The figure shows three views and two pictorial views of one solid part (mm, origin at its lowest corner). Answer the questions. A direction names the side the tool comes from. Give positions to 0.01 mm unless a question says otherwise; leave off trailing zeros. Loops run counter-clockwise (first coordinate to the right, second up) from the corner with the lowest first, then second, coordinate; pieces in that order, holes last. Notation, with made-up numbers: M -15.5,-20 L 12.5,-20 A15 ccw 12.5,4 Z; hole C 27,24.5 d1. An arc over 180 degrees is marked long. Answer in a Markdown table with one row per item. Add a question column.
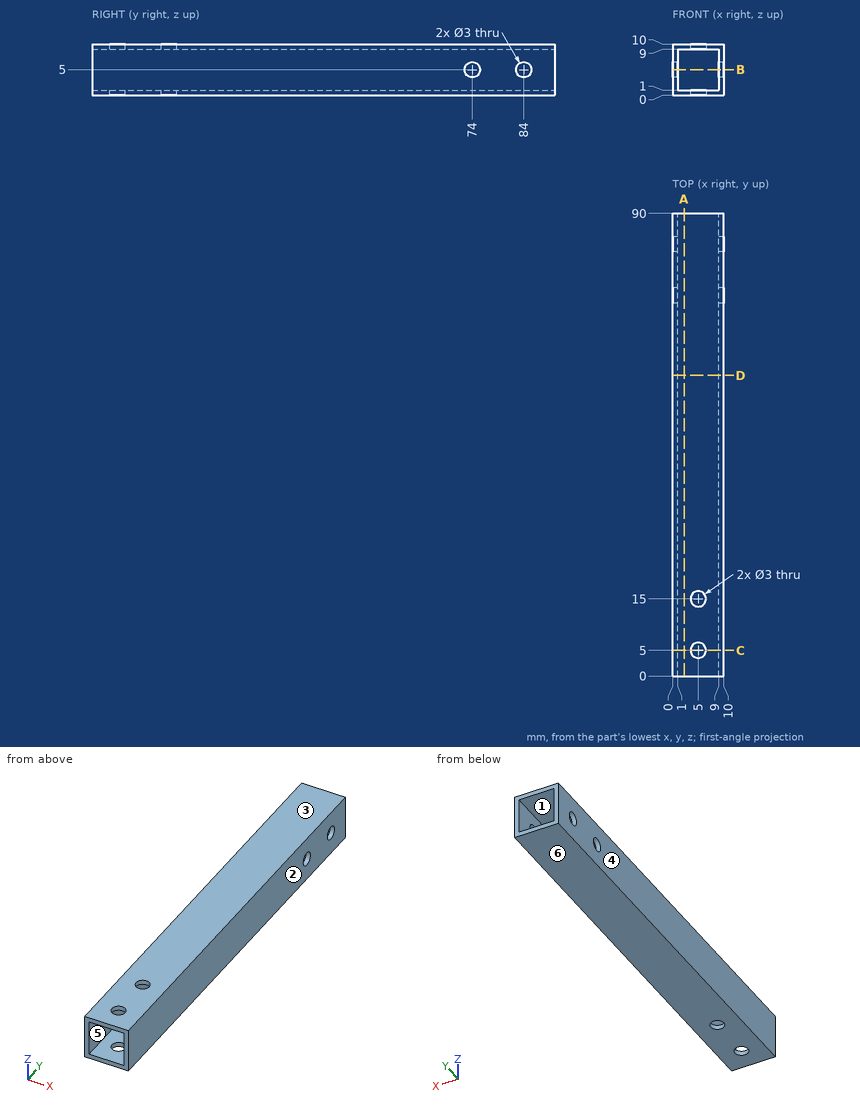
(1) Each of these flat-tipped pins is pushed along its axis until it touches: P1, Ø2.5, axis at x = 4, y = 30, coming from the -Z side; P2, Ø2.5, axis at y = 84, z = 5, coming from the +X side. Where does it stop, or does it pass through?
(2) Consider line 1 along Y through (x, z) = (5, 0.5); line 2 along Y through (x, z) = (9.5, 5); line 3 along Z through (x, y) = (9.2, 74). Determine where each line is inside the solid, lowest interval first. Write a range as from..to.
(3) Section A-A, the plane x = 2.25 is taken. Determine the outline of the cut face in (y, z).
(4) Section C-C, the plane y = 5 is taken. Determine the outline of the cut face in (x, z).
(5) The mould has two halves that part along Z. Classify the marked faces 3, 4, 5 and 6: pulls with the +Z half, pulls with the -Z half, needs draft (parallel to the pull), parting line crosses it, or undercut.
(6) Section D-D, the plane y = 58.5 is taken. Determine the outline of the cut face in (x, z).
(7) Which of the six approach directions +Z, -Z, +X, -X, +Y, -Y give full straight-line access (tool end or side, diameter ignored) to the marked faces 1 and 2?
(8) Section B-B, the plane z = 5 is taken. Determine the outline of the cut face in (x, y), and give its area (3 significant figures).
Numbers:
| question | item | result |
|---|---|---|
| 1 | P1 | stops at z = 0 |
| 1 | P2 | passes through |
| 2 | line 1 | y = 0..3.5, 6.5..13.5, 16.5..90 |
| 2 | line 2 | y = 0..72.5, 75.5..82.5, 85.5..90 |
| 2 | line 3 | z = 0..3.5, 6.5..10 |
| 3 | outline | M 0,0 L 90,0 L 90,1 L 0,1 Z; M 0,9 L 90,9 L 90,10 L 0,10 Z |
| 4 | outline | M 0,0 L 3.5,0 L 3.5,1 L 1,1 L 1,9 L 3.5,9 L 3.5,10 L 0,10 Z; M 6.5,0 L 10,0 L 10,10 L 6.5,10 L 6.5,9 L 9,9 L 9,1 L 6.5,1 Z |
| 5 | face 3 | pulls with the +Z half |
| 5 | face 4 | needs draft |
| 5 | face 5 | undercut |
| 5 | face 6 | pulls with the -Z half |
| 6 | outline | M 0,0 L 10,0 L 10,10 L 0,10 Z; hole M 1,1 L 9,1 L 9,9 L 1,9 Z |
| 7 | face 1 | +Y, -Y |
| 7 | face 2 | +Z, -Z, +X, +Y, -Y |
| 8 | outline | M 0,0 L 1,0 L 1,72.5 L 0,72.5 Z; M 0,75.5 L 1,75.5 L 1,82.5 L 0,82.5 Z; M 0,85.5 L 1,85.5 L 1,90 L 0,90 Z; M 9,0 L 10,0 L 10,72.5 L 9,72.5 Z; M 9,75.5 L 10,75.5 L 10,82.5 L 9,82.5 Z; M 9,85.5 L 10,85.5 L 10,90 L 9,90 Z |
| 8 | area | 168 mm² |
